Autodesk Inventor part; units mm, degrees
ref_plane "YZ Plane" through (0, 0, 0) normal (1, 0, 0) x (0, 1, 0)
ref_plane "XZ Plane" through (0, 0, 0) normal (0, 1, 0) x (-1, 0, 0)
ref_plane "XY Plane" through (0, 0, 0) normal (0, 0, 1) x (1, 0, 0)
sketch "Sketch1" plane through (0, 0, 0) normal (0, 0, 1) x (1, 0, 0)
  line L0 (-4, 9.5) -> (4, 9.5)
  line L1 (4, 9.5) -> (4, -9.5)
  line L2 (4, -9.5) -> (-4, -9.5)
  line L3 (-4, -9.5) -> (-4, 9.5)
  line L4 (-4, 9.5) -> (4, -9.5) construction
  line L5 (4, 9.5) -> (-4, -9.5) construction
  line L6 (4, 9.5) -> (8, 9.5)
  line L7 (8, 9.5) -> (8, 4.5)
  line L8 (8, 4.5) -> (4, 4.5)
  line L9 (4, 4.5) -> (4, 9.5)
  line L10 (8, -0.5) -> (4, -0.5)
  line L11 (8, 4.5) -> (8, -0.5)
  line L12 (8, -5.5) -> (4, -5.5)
  line L13 (8, -0.5) -> (8, -5.5)
  line L14 (2, 14.112) -> (2, 5.4586)
  line L15 (0, 9.5) -> (0, -9.5)
  line L16 (0, 9.5) -> (-4, 9.5)
  line L17 (-4, 9.5) -> (-4, 4.5)
  line L18 (-4, 4.5) -> (0, 4.5)
  line L19 (-4, -0.5) -> (0, -0.5)
  line L20 (-4, 4.5) -> (-4, -0.5)
  line L21 (-4, -0.5) -> (-4, -9.5)
  line L22 (-4, -5.5) -> (0, -5.5)
  line L23 (4, -5.5) -> (8, -5.5)
  line L24 (8, -5.5) -> (8, -9.5)
  line L25 (8, -9.5) -> (4, -9.5)
  line L26 (4, -9.5) -> (4, -5.5)
  point P0 (0, 0)
  point P1 (0, 4.5)
  point P2 (-4, 4.5)
  point P3 (-4, -0.5)
  point P4 (4, -7)
  point P5 (8, -0.5)
  point P6 (0, 9.5)
  point P7 (8, 4.5)
  point P8 (4, -5.5)
  point P9 (0, -5.5)
  point P10 (-4, -5.5)
  dimension "d0" = 8
  dimension "d1" = 19
  dimension "d2" = 4
  dimension "d3" = 5
  dimension "d6" = 5
  dimension "d11" = 12
  dimension "d12" = 6
extrude "Extrusion1" add sketch "Sketch1" along normal blind 4 contours L0 L1 L2 L15 | L18 L15 L19 L3 | L6 L7 L8 L1 | L22 L15 L2 L3 | L10 L13 L12 L1 | L12 L24 L25 L1
sketch "Sketch2" plane through (0, 0, 4) normal (0, 0, 1) x (1, 0, 0)
  line L0 (0, -5.5) -> (-4, -5.5)
  line L1 (-4, -5.5) -> (-4, -9.5)
  line L2 (-4, -9.5) -> (8, -9.5)
  line L3 (8, -9.5) -> (8, -0.5)
  line L4 (8, -0.5) -> (4, -0.5)
  line L5 (4, -0.5) -> (4, 4.5)
  line L6 (4, 4.5) -> (8, 4.5)
  line L7 (8, 4.5) -> (8, 9.5)
  line L8 (8, 9.5) -> (0, 9.5)
  line L9 (0, 9.5) -> (0, 4.5)
  line L10 (0, 4.5) -> (-4, 4.5)
  line L11 (-4, 4.5) -> (-4, -0.5)
  line L12 (-4, -0.5) -> (0, -0.5)
  line L13 (0, -0.5) -> (0, -5.5)
  point P0 (0, 0)
equation "\"d1\" = height + e"
equation "\"d2\" = e"
equation "\"d3\" = 0.333333 * height"
equation "\"d6\" = d3"
equation "\"d12\" = 0.5 * d11"
equation "\"d13\" = e"
equation "\"e\" = 4"
equation "\"height\" = 15"
properties part number "wall2" material "MDF Medium Density Fiberboard"
Source: CAD feature listing. Evaluate the final solid. Frame: model axes, mm. A direction names the side the tool comes from. Coordinates: 2 decimals unless noted, no trailing zeros. Loops run counter-clockwise (first coordinate to the right, second up) from the corner with the lowest first, then second, coordinate; pieces in that order, holes last. Notation, with made-up numbers: M -29.75,-19.75 L -14.75,-19.75 A22 ccw -14.75,4.25 Z; hole C -4.5,63.25 d4. An arc over 180 degrees is marked long. Use CSV: the item, a comma, the result in double quotes.
(1) Cut plane C-C on x = -2.5. Return loops of the section in (y, z), and give its area (3 significant figures).
Answers follow:
outline,"M -9.5,0 L -5.5,0 L -5.5,4 L -9.5,4 Z; M -0.5,0 L 4.5,0 L 4.5,4 L -0.5,4 Z"
area,"36.0 mm²"
(2) Line query: line 1 (Y direction, x = -1.25, z = 1.15); line 2 (Y direction, x = 6.75, z = 3.1); line 3 (X direction, y = 0, z = 0.9). Output: solid intervals per line, ascending. Write a range as [from, to].
Answers follow:
line 1,"[-9.5, -5.5], [-0.5, 4.5]"
line 2,"[-9.5, -0.5], [4.5, 9.5]"
line 3,"[-4, 4]"
(3) Draft query along Y for faces 1 (the face through (-2, 4.5, 2)), 2 (the face through (8, -5, 2)), 3 (the face through (0, -3, 2)). Return one class per face: pulls with the +Y half, pulls with the -Y half, needs draft (parallel to the pull), parting line crosses it, or undercut.
Answers follow:
face 1,"pulls with the +Y half"
face 2,"needs draft"
face 3,"undercut"
(4) Cut plane D-D on y = 6.75. Return loops of the section in (x, z).
Answers follow:
outline,"M 0,0 L 8,0 L 8,4 L 0,4 Z"
(5) Cut plane B-B on z = 1.95. Return loops of the section in (x, y), and give its area (3 significant figures).
Answers follow:
outline,"M -4,-9.5 L 8,-9.5 L 8,-0.5 L 4,-0.5 L 4,4.5 L 8,4.5 L 8,9.5 L 0,9.5 L 0,4.5 L -4,4.5 L -4,-0.5 L 0,-0.5 L 0,-5.5 L -4,-5.5 Z"
area,"168 mm²"
(6) Cut plane A-A on x = 4.5. Return loops of the section in (y, z), and give its area (3 significant figures).
Answers follow:
outline,"M -9.5,0 L -0.5,0 L -0.5,4 L -9.5,4 Z; M 4.5,0 L 9.5,0 L 9.5,4 L 4.5,4 Z"
area,"56.0 mm²"
(7) Reachability of faces 4 (the face through (2, -9.5, 2)), 5 (the face through (-4, 2, 2)), 6 (the face through (0, 7, 2)), 7 (the face through (6, 4.5, 2)), 8 (the face through (-2, -5.5, 2)) from +Z, -Z, +X, -X, +Y, -Y: full face, straight path, thin tool, end or side. Return the list, or none.
Answers follow:
face 4,"+Z, -Z, +X, -X, -Y"
face 5,"+Z, -Z, -X, +Y, -Y"
face 6,"+Z, -Z, -X, +Y"
face 7,"+Z, -Z, +X"
face 8,"+Z, -Z, -X"
(8) Contact query for flat-ended pins moving along their axis: pin 1 (2 mm diameter, centred on y = 7, z = 2.5, fed in from -X); pin 2 (2 mm diameter, centred on y = 1.5, z = 1.5, fed in from +X); pin 3 (1.2 mm diameter, centred on x = -1.5, z = 2.5, fed in from +Y). Output: stop coordinate, or through.
Answers follow:
pin 1,"x = 0"
pin 2,"x = 4"
pin 3,"y = 4.5"
